Source: CAD feature listing. Evaluate the final solid. Frame: model axes, mm. A direction names the side the tool comes from. Coordinates: 2 decimals unless noted, no trailing zeros. Write each loop counter-clockwise with the first axis right and the second up, starting at its lowest first coordinate (ties: lowest second). Pieces come first, ordered by that corner, then holes. Notation, with made-up numbers: (-7, 8) - (39, 8) arc R17 ccw to (39, 31) - close; hole circle Ø1 at (33.25, 76). An arc over 180 degrees is marked (long way). One line per question, with ' | ' between items. Start each with the question number.
Q1. Draft query along Y for faces 3 (the face through (-2, 0, 38)), 4 (the face through (-23, 123, 50)), 5 (the face through (-32.92, -10.32, 31.41)), 6 (the face through (-17.143, 79.994, 12.675)). Return one class per face: +Y half, -Y half, draft (parallel to the pull), parting line (faces both ways), or undercut.
Q2. Line query: line 1 (Y direction, x = 0, z = 31.75); line 2 (X direction, y = 0, z = 33.5); line 3 (Y direction, x = -20, z = 32.5). Output: solid intervals per line, ascending.
Q3. Cut plane B-B, the plane y = 63. Return loops of the section in (x, z), plus the area to 3 significant figures.
Q4. Cut plane A-A, the plane y = 0. Return loops of the section in (x, z), plus the area to 3 significant figures.
Q5. Contact query for flat-ended pins moving along their axis: P1, Ø2, axis at y = 141.5, z = 15.5, coming from the -X side; P2, Ø2, axis at y = 161.5, z = 28.5, coming from the +X side; P3, Ø25, axis at y = 19.5, z = 15.5, coming from the -X side. Output: stop coordinate, or through.
Q6. Access query for faces 1 (the face through (-35, 31, 36)), 2 (the face through (-45, 181, 0)). Directions: +Z, -Z, +X, -X, +Y, -Y. A direction counts if a zero-diameter tool reaches every point of the face in a straight line with its end or side. Return the directions, or none.
```python
from build123d import *

# Parameters (mm, degrees)
BOSS_EXTRUDE1_DEPTH = 50
SKETCH3_W           = 66.376369139
SKETCH3_H           = 188.96079622
CUT_EXTRUDE1_DEPTH  = 305.408240944
SKETCH4_R           = 34.5
CUT_EXTRUDE2_DEPTH  = 13
CUT_EXTRUDE3_DEPTH  = 300.667940806


with BuildPart() as part:
    # Sketch1 → Boss-Extrude1 (new body)
    with BuildSketch(Plane.XY):
        with BuildLine():
            Line((0.221790001, 84.828286355), (0.2207262, 284.828286352))
            add(Edge.make_bspline(
                [(0.2207262, 284.828286352), (-159.978737061, 262.606607754), (-63.000724603, 150.139017081), (-35, 85.625)],
                knots=[0, 0, 0, 0, 1, 1, 1, 1], degree=3))
            Line((-35, 85.625), (-35, -85.625))
            Line((-35, -85.625), (35, -85.625))
            Line((35, -85.625), (35, -40.1019375))
            Line((35, -40.1019375), (0.221790001, 84.828286355))
        make_face()
    extrude(amount=BOSS_EXTRUDE1_DEPTH)

    # Sketch3 → Cut-Extrude1 (cut, through all)
    with BuildSketch(Plane(origin=(22.122011617, 6.158349372, 0), x_dir=(0, 0, -1), z_dir=(0.9633678796634119, 0.2681833858254875, 0))):
        with Locations((8.18818457, -12.819032142)):
            Rectangle(SKETCH3_W, SKETCH3_H)
    extrude(amount=-CUT_EXTRUDE1_DEPTH, mode=Mode.SUBTRACT)

    # Sketch4 → Cut-Extrude2 (cut)
    with BuildSketch(Plane(origin=(0, 0, 25), x_dir=(-1, 0, 0), z_dir=(0, 0, -1))):
        Circle(SKETCH4_R)
    extrude(amount=-CUT_EXTRUDE2_DEPTH, mode=Mode.SUBTRACT)

    # Sketch5 → Cut-Extrude3 (cut, through all)
    with BuildSketch(Plane(origin=(0, 0, 25), x_dir=(-1, 0, 0), z_dir=(0, 0, -1))):
        with BuildLine():
            Line((35, -40.1019375), (35, -85.625))
            Line((35, -85.625), (-35, -85.625))
            Line((-35, -85.625), (-35, -40.1019375))
            Line((-35, -40.1019375), (-32.013551407, -29.374022196))
            ThreePointArc((-32.013551407, -29.374022196), (2.35071235, -43.384038598), (35, -25.742972899))
            Line((35, -25.742972899), (35, -40.1019375))
        make_face()
    extrude(amount=-CUT_EXTRUDE3_DEPTH, mode=Mode.SUBTRACT)


solid = part.part
```
Reply:
1) face 3: undercut | face 4: draft | face 5: undercut | face 6: -Y half
2) line 1: y = -43.45 to -34.5, 34.5 to 284.8 | line 2: x = -35 to -34.5 | line 3: y = -38.57 to -28.11, 28.11 to 281.27
3) outline: (-35, 25) - (6.3, 25) - (6.3, 50) - (-35, 50) - close | area: 1,030 mm^2
4) outline: (-35, 25) - (-34.5, 25) - (-34.5, 38) - (23.84, 38) - (23.84, 50) - (-35, 50) - close | area: 713 mm^2
5) P1: stops at x = -64.71 | P2: stops at x = 0.22 | P3: stops at x = -35
6) face 1: +Z, -Z, -X, -Y | face 2: -Z, +X, -X, +Y, -Y
